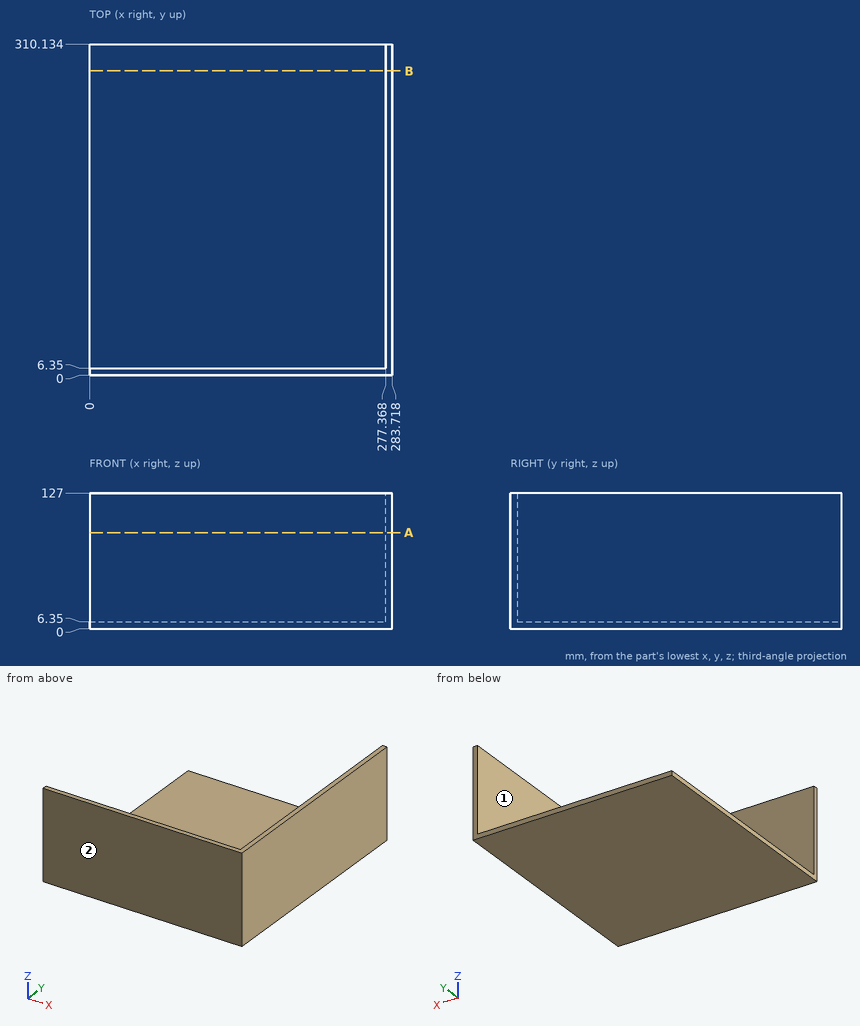
Here's the drawing with two shaded views (mm, measured from the low corner). I have some questions. A direction names the side the tool comes from. Give positions to 0.01 mm unless a question says otherwise; leave off trailing zeros. Write each loop counter-clockwise with the first axis right and the second up, starting at its lowest first coordinate (ties: lowest second). Pieces come first, ordered by that corner, then holes. Notation, with made-up numbers: (40.5, 52.25) -> (75.5, 52.25) arc R26 cw to (75.5, 80.25) -> close; hole circle Ø8 at (21, 2.25). An arc over 180 degrees is marked (long way). Use one line per item in the form item = value. Start each with the question number.
1. Imagine slicing it at A-A on z = 90. List the corners of the cut face in (x, y) for me.
2. Will these pins go through, and if not, where does the flat tip stop? pin 1 Ø10 at (y, z) = (250, 60) entering from -X; pin 2 Ø6 at (x, y) = (38.5, 195.5) entering from +Z.
3. On a 3-axis mill with a long thin cutter (end or side, diameter ignored), from which of +Z, -Z, +X, -X, +Y, -Y can I reach the whole of each face in a straight line? I mean the marked faces 1 and 2. Say none if no direction works.
4. If I drill on L1, parallel to Z at x = 154, y = 21; L2, parallel to X at y = 246.5, z = 102.5, over which ranges is the centre line in solid material (lowest first)?
5. Imagine slicing it at B-B on y = 285. List the corners of the cut face in (x, z) for me, plus the area to 3 significant figures.
Entries:
q1.outline = (0, 0) -> (283.72, 0) -> (283.72, 310.13) -> (277.37, 310.13) -> (277.37, 6.35) -> (0, 6.35) -> close
q2.pin_1 = 277.37
q2.pin_2 = 6.35
q3.face_1 = +Z, -X, +Y
q3.face_2 = +Z, -Z, +X, -X, -Y
q4.L1 = 0 to 6.35
q4.L2 = 277.37 to 283.72
q5.outline = (0, 0) -> (283.72, 0) -> (283.72, 127) -> (277.37, 127) -> (277.37, 6.35) -> (0, 6.35) -> close
q5.area = 2,570 mm²
